Verification items for this drawing (mm, ordinates from the low corner). Give positions to 0.01 mm unless a question says otherwise; leave off trailing zeros. Loops run counter-clockwise (first coordinate to the right, second up) from the corner with the lowest first, then second, coordinate; pieces in that order, holes last. Notation, with made-up numbers: (75.5, 29) -> (94.5, 29) arc R25 cw to (94.5, 41) -> close; hole circle Ø6 at (22.25, 23). An arc over 180 degrees is marked (long way). Write each question's results on one line, items separated by ' | '. Start each with the question number.
1) Sectioned sample at B-B on z = 1.6. Count the separate pieces of the cut face and the enclosed holes in it, then the cut area to 3 significant figures.
2) Sectioned sample at D-D on x = 47. Record the cut outline in (y, z).
3) Scan lines: line 1 (Y direction, x = 8, z = 1.6); line 2 (Y direction, x = 64.5, z = 2.05); line 3 (X direction, y = 14.5, z = 2.65). Record each from-to range of solid material in increasing order. Write a range as from..to.
4) Sectioned sample at C-C on y = 11.5. Record the cut outline in (x, z).
5) Sectioned sample at A-A on x = 8. Record the cut outline in (y, z).
6) Depth check by flat-ended pin: pin 1 (1 mm diameter, centred on x = 26, z = 2.5, fed in from -Y); pin 2 (2.5 mm diameter, centred on x = 62, y = 20.59, fed in from +Z). Enter the tip coordinate at first touch or a pass-through.
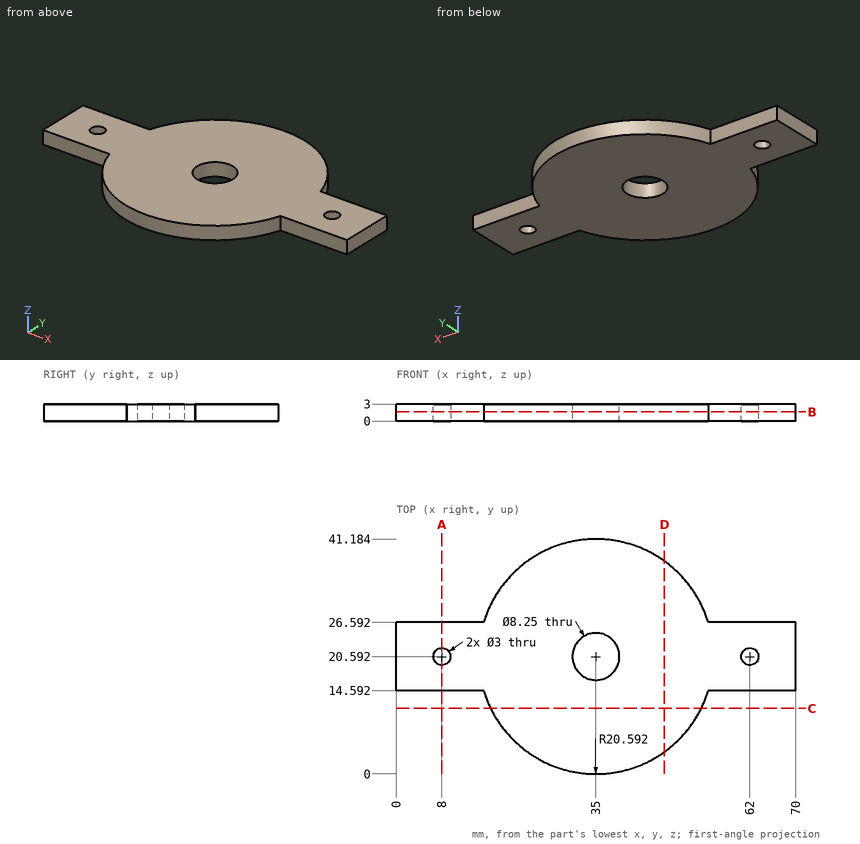
Result:
1) separate pieces: 1 | enclosed holes: 3 | area: 1,620 mm^2
2) outline: (3.86, 0) -> (37.33, 0) -> (37.33, 3) -> (3.86, 3) -> close
3) line 1: 14.59..19.09, 22.09..26.59 | line 2: 14.59..26.59 | line 3: 15.33..54.67
4) outline: (16.52, 0) -> (53.48, 0) -> (53.48, 3) -> (16.52, 3) -> close
5) outline: (14.59, 0) -> (19.09, 0) -> (19.09, 3) -> (14.59, 3) -> close; (22.09, 0) -> (26.59, 0) -> (26.59, 3) -> (22.09, 3) -> close
6) pin 1: y = 1.84 | pin 2: through
